Verification items for this drawing (mm, ordinates from the low corner). Give positions to 0.01 mm unless a question says otherwise; leave off trailing zeros. Loops run counter-clockwise (first coordinate to the right, second up) from the corner with the lowest first, then second, coordinate; pieces in that order, holes last. Notation, with made-up numbers: M -30.75,60 L -19.75,60 A26 cw -19.75,83 Z; hole C 50.5,44 d2. An arc over 180 degrees is marked long. Answer in a Markdown table with one row per item.
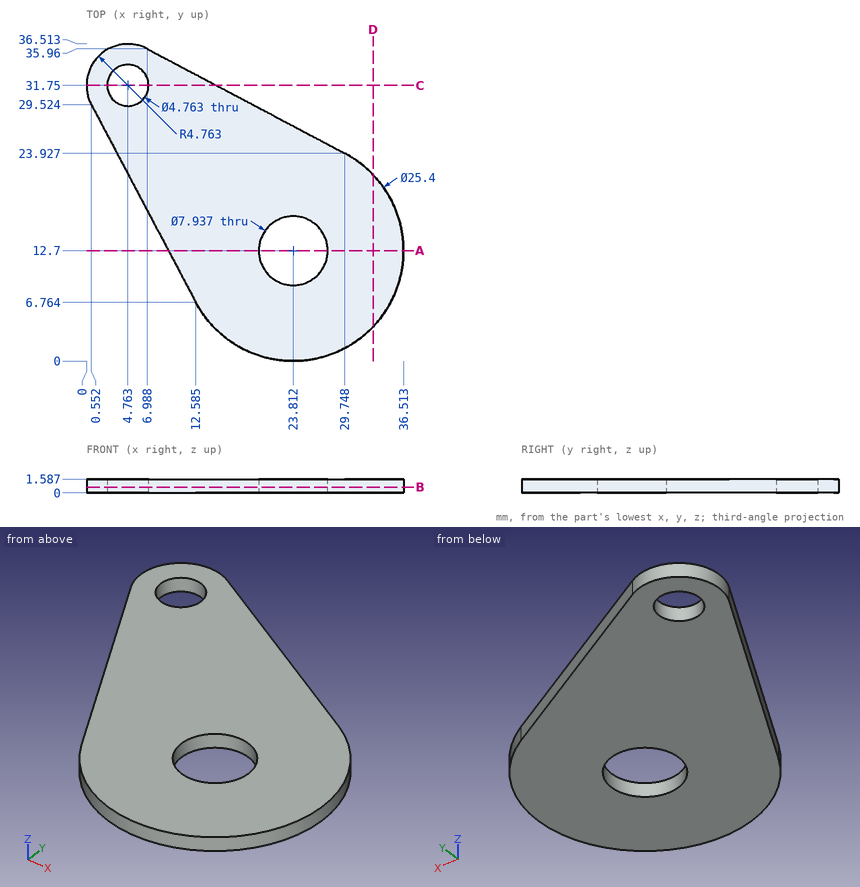
Item 1: Scan lines: L1, parallel to Y at x = 16.5, z = 1.1 (1 decimal); L2, parallel to X at y = 15, z = 0.85 (1 decimal); L3, parallel to Y at x = 20.5, z = 0.2 (1 decimal). Record each from-to range of solid material in increasing order. Write a range as [from, to].
Reported:
| item | result |
|---|---|
| L1 | y = [2.3, 30.9] |
| L2 | x = [8.2, 20.6], [27, 36.3] |
| L3 | y = [0.4, 10.5], [14.9, 28.8] |
Item 2: Sectioned sample at D-D (x = 33). Record the cut outline in (y, z).
Reported:
| item | result |
|---|---|
| outline | M 3.93,0 L 21.47,0 L 21.47,1.59 L 3.93,1.59 Z |
Item 3: Sectioned sample at C-C (y = 31.75). Record the cut outline in (x, z).
Reported:
| item | result |
|---|---|
| outline | M 0,0 L 2.38,0 L 2.38,1.59 L 0,1.59 Z; M 7.14,0 L 14.95,0 L 14.95,1.59 L 7.14,1.59 Z |
Item 4: Sectioned sample at B-B (z = 0.65). State how many separate pieces and enclosed holes the cut face has, and give its area (3 significant figures).
Reported:
| item | result |
|---|---|
| separate pieces | 1 |
| enclosed holes | 2 |
| area | 713 mm^2 |
Item 5: Sectioned sample at A-A (y = 12.7). Record the cut outline in (x, z).
Reported:
| item | result |
|---|---|
| outline | M 9.45,0 L 19.84,0 L 19.84,1.59 L 9.45,1.59 Z; M 27.78,0 L 36.51,0 L 36.51,1.59 L 27.78,1.59 Z |
